CAD build for the part. Positions are in the model's coordinates, mm. A direction names the side the tool comes from. Coordinates: 2 decimals unless noted, no trailing zeros. Loops run counter-clockwise (first coordinate to the right, second up) from the corner with the lowest first, then second, coordinate; pieces in that order, holes last. Notation, with made-up numbers: (48.25, 22) -> (106.25, 22) arc R27 cw to (106.25, 61) -> close; hole circle Ø5 at (36, 67). An arc over 180 degrees is marked (long way). Return JSON: item names as keys, results as strings. Group by question number.
(1) Saw through at C-C on y = 1.75. Write the cut outline in (x, z), then the cut area to 3 significant figures.
(2) Saw through at A-A on y = 7.41. Write the cut outline in (x, z).
(3) Saw through at D-D on z = -12.5. Write the cut outline in (x, y).
(4) Probe L1, parallel to Y at x = -8.51, z = 0.45; L2, parallel to Z at x = -7, y = 8.5; L3, parallel to Z at x = -6.5, y = -0.25. List the from-to ranges inside material, lowest first.
(5) Tool access for faces 1 (the face through (6, -7.41, 6)), 2 (the face through (9.46, -4, 6)), 3 (the face through (-2.6, -6.5, 0)): list every direction of +Z, -Z, +X, -X, +Y, -Y with a clear straight run to the whole face (end or side of a thin tool).
(6) Saw through at B-B on x = -1.25. Write the cut outline in (y, z).
(7) Flat gauge pins, fed straight in: pin 1 Ø8 at (x, y) = (-8.5, 7) entering from +Z; pin 2 Ø1 at (x, z) = (1.5, 6.5) entering from +Y; pin 3 Ø6 at (y, z) = (-5.5, 7.5) entering from -X. Where does each tip first touch, or does it go through?
(8) Mould opens along Y. For faces 4 (the face through (-0.2, -9.95, 0.4)), 5 (the face through (-7.032, -6.944, 0.444)), 6 (the face through (1.07, 9.88, -7.2)), 7 (the face through (9.34, 8.72, 0.44)) say: pulls with the +Y half, pulls with the -Y half, needs draft (parallel to the pull), parting line crosses it, or undercut.
```python
from build123d import *

# Parameters (mm, degrees)
SKETCH2_W           = 22.1
SKETCH2_H           = 19.9
SKETCH2_R           = 1.55
BOSS_EXTRUDE1_DEPTH = 0.9
SKETCH3_W           = 7.5
SKETCH3_H           = 7.62
BOSS_EXTRUDE2_DEPTH = 9.525
SKETCH4_R           = 8.2
BOSS_EXTRUDE3_DEPTH = 14.6


with BuildPart() as part:
    # Sketch2 → Boss-Extrude1 (new body)
    with BuildSketch(Plane.XY):
        Rectangle(SKETCH2_W, SKETCH2_H)
        with Locations((-8.51, -7.41)):
            Circle(SKETCH2_R, mode=Mode.SUBTRACT)
        with Locations((8.51, 7.41)):
            Circle(SKETCH2_R, mode=Mode.SUBTRACT)
    extrude(amount=BOSS_EXTRUDE1_DEPTH)

    # Sketch3 → Boss-Extrude2 (add)
    with BuildSketch(Plane.XY.offset(0.9)):
        with Locations((5.710174181, -3.6)):
            Rectangle(SKETCH3_W, SKETCH3_H)
    extrude(amount=BOSS_EXTRUDE2_DEPTH)

    # Sketch4 → Boss-Extrude3 (add)
    with BuildSketch(Plane(origin=(0, 0, 0), x_dir=(-1, 0, 0), z_dir=(0, 0, -1))):
        with Locations((0, 1.75)):
            Circle(SKETCH4_R)
    extrude(amount=BOSS_EXTRUDE3_DEPTH)


solid = part.part
```
Geometry results:
{
 "1": {"outline": "(-11.05, 0) -> (-8.2, 0) -> (-8.2, -14.6) -> (8.2, -14.6) -> (8.2, 0) -> (11.05, 0) -> (11.05, 0.9) -> (-11.05, 0.9) -> close", "area": "259 mm²"},
 "2": {"outline": "(-11.05, 0) -> (-5.93, 0) -> (-5.93, -14.6) -> (5.93, -14.6) -> (5.93, 0) -> (6.96, 0) -> (6.96, 0.9) -> (-11.05, 0.9) -> close; (10.06, 0) -> (11.05, 0) -> (11.05, 0.9) -> (10.06, 0.9) -> close"},
 "3": {"outline": "circle Ø16.4 at (0, 1.75)"},
 "4": {"L1": "-9.95 to -8.96, -5.86 to 9.95", "L2": "0 to 0.9", "L3": "-14.6 to 0.9"},
 "5": {"face 1": "+Z, +X, -X, -Y", "face 2": "+Z, +X, +Y, -Y", "face 3": "-Z"},
 "6": {"outline": "(-9.95, 0) -> (-6.35, 0) -> (-6.35, -14.6) -> (9.85, -14.6) -> (9.85, 0) -> (9.95, 0) -> (9.95, 0.9) -> (-9.95, 0.9) -> close"},
 "7": {"pin 1": "z = 0.9", "pin 2": "y = 0.21", "pin 3": "x = 1.96"},
 "8": {"face 4": "pulls with the -Y half", "face 5": "undercut", "face 6": "parting line crosses it", "face 7": "undercut"}
}
